CAD build for the part. Positions are in the model's coordinates, mm. Round coordinates to 2 decimals unless told otherwise and drop trailing zeros. Order: outer loops, then holes, each group sorted by start corner. A loop starts at its lowest first (then second) coordinate and runs counter-clockwise, first axis right, second up. Notation, with made-up numbers: M -33,-8 L -2,-8 A24 ccw -2,11 Z; hole C 40,-22 d11. An arc over 180 degrees is marked long. Put each result on its own line as item: value.
Autodesk Fusion 360 part; units mm, degrees
sketch "Sketch1" plane through (0, 0, 0) normal (0, 0, 1) x (1, 0, 0)
  line L0 (10, -35) -> (-10, -35)
  line L1 (-10, -35) -> (-10, 35)
  line L2 (-10, 35) -> (10, 35)
  line L3 (10, 35) -> (10, -35)
  line L4 (10, -35) -> (-10, 35) construction
  line L5 (-10, -35) -> (10, 35) construction
  line L6 (10, 35) -> (0, 35)
  line L7 (0, 35) -> (0, 25)
  line L8 (0, 25) -> (10, 25)
  line L9 (10, 25) -> (10, 35)
  line L10 (0, 25) -> (0, -15)
  circle A0 centre (0, -15) radius 2
  circle A1 centre (0, 25) radius 2.5
  dimension "d1" = 20
  dimension "d2" = 70
  dimension "d3" = 10
  dimension "d4" = 10
  dimension "d5" = 40
  dimension "d25" = 4
  dimension "d26" = 5
extrude "Extrude1" add sketch "Sketch1" against normal blind 2 contours A0 | L0 L1 L2 L3 L7 L8 A1 | L2 L3 L6 L7 L8 L9 A1 | L8 L10 A1 | L7 L8 A1 | L7 L10 A1
hole "Hole1" at (0, 25, 0) direction (0, 0, -1) diameter 4.234 depth 3 tip angle 118
sketch "Sketch2" plane through (0, 0, 0) normal (0, 0, 1) x (1, 0, 0)
  line L0 (2.2126, 24.4763) -> (7.2126, 24.4763) construction
  line L1 (7.2126, 24.4763) -> (7.2126, 28.4763) construction
  line L2 (7.2126, 28.4763) -> (2.2126, 28.4763) construction
  line L3 (2.2126, 28.4763) -> (2.2126, 24.4763) construction
  dimension "d18" = 2
  dimension "d19" = 0
hole "Hole3" at (0, -15, 0) direction (0, 0, -1) diameter 4 depth 20 tip angle 118
equation "d19 = 'M5'"
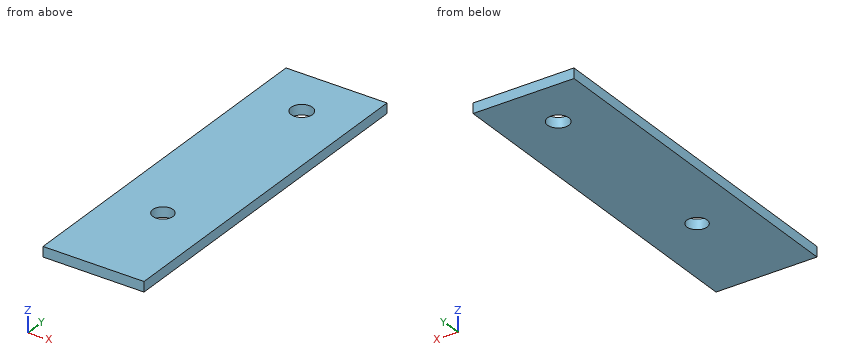
Item 1: Band-saw the part on C-C on z = -1.3. Give the cut face in (x, y), and give its area (3 significant figures).
Answers below:
outline: M -10,-35 L 10,-35 L 10,35 L -10,35 Z; hole C 0,25 d4.23; hole C 0,-15 d4
area: 1,370 mm²
Item 2: Probe line 1 along Y through (x, z) = (0, -1.2); line 2 along X through (y, z) = (25, -0.7); line 3 along Y through (x, z) = (1, -0.85). List the from-to ranges inside material, lowest first. Write a range as [from, to].
Answers below:
line 1: [-35, -17], [-13, 22.88], [27.12, 35]
line 2: [-10, -2.12], [2.12, 10]
line 3: [-35, -16.73], [-13.27, 23.13], [26.87, 35]
Item 3: Band-saw the part on A-A on y = -15. Give the cut face in (x, z), and give its area (3 significant figures).
Answers below:
outline: M -10,-2 L -2,-2 L -2,0 L -10,0 Z; M 2,-2 L 10,-2 L 10,0 L 2,0 Z
area: 32.0 mm²
Item 4: Band-saw the part on B-B on y = 25. Give the cut face in (x, z).
Answers below:
outline: M -10,-2 L -2.12,-2 L -2.12,0 L -10,0 Z; M 2.12,-2 L 10,-2 L 10,0 L 2.12,0 Z
Item 5: Pin check, flat tips, straight feed: P1, Ø10, axis at x = 3, y = 9.5, coming from the +Z side; P2, Ø2.5, axis at x = 0, y = 25, coming from the -Z side. Stop position of each tip, or through.
Answers below:
P1: z = 0
P2: through
